```python
from build123d import *

# Parameters (mm, degrees)
SKETCH1_R               = 15
SKETCH1_R_2             = 3
BOSS_EXTRUDE1_DEPTH     = 10
SKETCH2_W               = 15
SKETCH2_H               = 30
BOSS_EXTRUDE2_DEPTH     = 10
FILLET1_R               = 15
SKETCH5_W               = 10
SKETCH5_H               = 2
BOSS_EXTRUDE3_DEPTH     = 10
BOSS_EXTRUDE4_START     = -3
SKETCH7_R               = 3
BOSS_EXTRUDE4_DEPTH     = 3
CHAMFER1_SIZE           = 0.7
BOSS_EXTRUDE6_DEPTH     = 10
FILLET4_R               = 2
FILLET2_R               = 10
CUT_EXTRUDE1_DEPTH      = 63.556116013
CUT_EXTRUDE1_DEPTH_BACK = 63.556116013
SKETCH10_R              = 1.25


with BuildPart() as part:
    # Sketch1 → Boss-Extrude1 (new body)
    with BuildSketch(Plane.XY):
        Circle(SKETCH1_R)
        Circle(SKETCH1_R_2, mode=Mode.SUBTRACT)
    extrude(amount=BOSS_EXTRUDE1_DEPTH)

    # Sketch2 → Boss-Extrude2 (add)
    with BuildSketch(Plane.XY):
        with Locations((0, 27.990381057)):
            Rectangle(SKETCH2_W, SKETCH2_H)
    extrude(amount=BOSS_EXTRUDE2_DEPTH)

    # Fillet1
    fillet1_edges = [part.edges().sort_by_distance(p)[0] for p in [
        (-7.5, 12.990381057, 5),
        (7.5, 12.990381057, 5),
    ]]
    fillet(fillet1_edges, radius=FILLET1_R)

    # Sketch5 → Boss-Extrude3 (add)
    with BuildSketch(Plane(origin=(0, 0, 0), x_dir=(-1, 0, 0), z_dir=(0, 0, -1))):
        with Locations((0, 2.5)):
            Rectangle(SKETCH5_W, SKETCH5_H)
    extrude(amount=-BOSS_EXTRUDE3_DEPTH)

    # Sketch7 → Boss-Extrude4 (add)
    with BuildSketch(Plane.XY.offset(10).offset(BOSS_EXTRUDE4_START)):
        Circle(SKETCH7_R)
    extrude(amount=BOSS_EXTRUDE4_DEPTH)

    # Chamfer1
    chamfer1_edges = [part.edges().sort_by_distance(p)[0] for p in [
        (0, 1.5, 7),
        (0, -3, 7),
    ]]
    chamfer(chamfer1_edges, length=CHAMFER1_SIZE)

    # Sketch9 → Boss-Extrude6 (add)
    with BuildSketch(Plane(origin=(0, 0, 0), x_dir=(-1, 0, 0), z_dir=(0, 0, -1))):
        with BuildLine():
            Line((-15, 53.990381057), (-15, 50.490381057))
            ThreePointArc((-15, 50.490381057), (-12.803300859, 45.187080198), (-7.5, 42.990381057))
            Line((-7.5, 42.990381057), (0, 42.990381057))
            Line((0, 42.990381057), (0, 46.490381057))
            Line((0, 46.490381057), (-7.5, 46.490381057))
            ThreePointArc((-7.5, 46.490381057), (-10.328427125, 47.661953932), (-11.5, 50.490381057))
            Line((-11.5, 50.490381057), (-11.5, 53.990381057))
            Line((-11.5, 53.990381057), (-15, 53.990381057))
        make_face()
        with BuildLine():
            Line((0, 46.490381057), (0, 42.990381057))
            Line((0, 42.990381057), (7.5, 42.990381057))
            ThreePointArc((7.5, 42.990381057), (12.803300859, 45.187080198), (15, 50.490381057))
            Line((15, 50.490381057), (15, 53.990381057))
            Line((15, 53.990381057), (11.5, 53.990381057))
            Line((11.5, 53.990381057), (11.5, 50.490381057))
            ThreePointArc((11.5, 50.490381057), (10.328427125, 47.661953932), (7.5, 46.490381057))
            Line((7.5, 46.490381057), (0, 46.490381057))
        make_face()
    extrude(amount=-BOSS_EXTRUDE6_DEPTH)

    # Fillet4
    # the kernel refuses this fillet: 2 mm, written as the material it takes off along each edge
    with BuildSketch(Plane(origin=(11.5, 53.990381057, -5), x_dir=(0, -1, 0), z_dir=(0, 0, 1)), Plane(origin=(15, 53.990381057, -5), x_dir=(-1, 0, 0), z_dir=(0, 0, 1)), Plane(origin=(-11.5, 53.990381057, -5), x_dir=(-1, 0, 0), z_dir=(0, 0, 1)), Plane(origin=(-15, 53.990381057, -5), x_dir=(0, -1, 0), z_dir=(0, 0, 1))) as fillet4_piece_1:
        with BuildLine():
            CenterArc((FILLET4_R, FILLET4_R), FILLET4_R, 180, 90)
            Line((0, FILLET4_R), (0, 0))
            Line((0, 0), (FILLET4_R, 0))
        make_face()
    extrude(amount=20, mode=Mode.SUBTRACT)

    # Fillet2
    fillet2_edges = [part.edges().sort_by_distance(p)[0] for p in [
        (-7.5, 42.990381057, 5),
        (7.5, 42.990381057, 5),
    ]]
    fillet(fillet2_edges, radius=FILLET2_R)

    # Sketch10 → Cut-Extrude1 (cut, two sides: drawn at the far end of the back side and taken through both)
    with BuildSketch(Plane(origin=(15, 0, 0), x_dir=(0, 0, -1), z_dir=(1, 0, 0)).offset(-CUT_EXTRUDE1_DEPTH_BACK)):
        with Locations((-5, 50.490381057)):
            Circle(SKETCH10_R)
    extrude(amount=CUT_EXTRUDE1_DEPTH + CUT_EXTRUDE1_DEPTH_BACK, mode=Mode.SUBTRACT)


solid = part.part
```
CAD build for the part. Positions are in the model's coordinates, mm. A direction names the side the tool comes from. Round coordinates to 2 decimals unless told otherwise and drop trailing zeros. Loops run counter-clockwise (first coordinate to the right, second up) from the corner with the lowest first, then second, coordinate; pieces in that order, holes last. Notation, with made-up numbers: M 50,-38 L 61,-38 A24 ccw 61,-14 Z; hole C -24,33 d10. An arc over 180 degrees is marked long. Use a Markdown table: item, result. Add a question column.
(1) Cut at C-C (y = 0). Give the cut face in (x, z).
(2) Cut at D-D (x = 0). Give the cut face in (y, z), and give its area (3 significant figures).
(3) Cut at B-B (x = 10.5). Give the cut face in (y, z).
(4) Cut at A-A (z = 2.75). Give the cut face in (x, y).
(5) Drill centre lines: line 1 (X direction, y = 50.5, z = 2.25); line 2 (Y direction, x = -13.65, z = 5); line 3 (Y direction, x = -13.85, z = 5). Where is each one in solid material? Low to high.
(6) Pull direction Y, two halves, no side cores. Call faces 1 (the face through (0, 46.49, 5)), 2 (the face through (0, 0, 7)), 3 (the face through (0, 12, 10)): +Y half, -Y half, draft (parallel to the pull), parting line (faces both ways), or undercut.
(7) Flat gauge pins, fed straight in: pin 1 (4 mm diameter, centred on x = -1, z = 4.5, fed in from -Y); pin 2 (2 mm diameter, centred on y = 50.49, z = 5, fed in from -X); pin 3 (1 mm diameter, centred on y = 20.5, z = 5, fed in from -X). Where does each tip first touch, or does it go through?
(8) Which spindle directions (+Z, -Z, +X, -X, +Y, -Y) get a long thin tool onto all of the face, cutting with end or side? Do faces 4 (the face through (0, 1.5, 3)), 5 (the face through (8.67, 40.82, 5.07)), 6 (the face through (-7.5, 28, 5)), 7 (the face through (10.297, 47.631, 4.93)). Say none if no direction does.
Geometry says:
| question | item | result |
|---|---|---|
| 1 | outline | M -15,0 L -3,0 L -3,6.3 L -2.3,7 L 2.3,7 L 3,6.3 L 3,0 L 15,0 L 15,10 L -15,10 Z |
| 2 | outline | M -15,0 L -3,0 L -3,6.3 L -2.3,7 L 0.8,7 L 1.5,6.3 L 1.5,0 L 46.49,0 L 46.49,10 L -15,10 Z |
| 2 | area | 584 mm² |
| 3 | outline | M -10.71,0 L 10.84,0 L 10.84,10 L -10.71,10 Z; M 43.27,0 L 47.84,0 L 47.84,10 L 43.27,10 Z |
| 4 | outline | M -15,50.49 A7.5 ccw -11.79,44.34 A10 cw -7.5,36.13 L -7.5,19.84 A15 cw -11.25,9.92 A15 ccw long 11.25,9.92 A15 cw 7.5,19.84 L 7.5,36.13 A10 cw 11.79,44.34 A7.5 ccw 15,50.49 L 15,51.99 A2 ccw 13.25,53.97 A2 ccw 11.5,51.99 L 11.5,50.49 A4 cw 7.5,46.49 L -7.5,46.49 A4 cw -11.5,50.49 L -11.5,51.99 A2 ccw -13.25,53.97 A2 ccw -15,51.99 Z; hole M -2.6,1.5 A3 ccw long 2.6,1.5 Z |
| 5 | line 1 | x = -15 to -11.5, 11.5 to 15 |
| 5 | line 2 | y = -6.22 to 6.22, 46.2 to 49.24, 51.74 to 53.88 |
| 5 | line 3 | y = -5.76 to 5.76, 46.5 to 49.24, 51.74 to 53.8 |
| 6 | face 1 | +Y half |
| 6 | face 2 | undercut |
| 6 | face 3 | draft |
| 7 | pin 1 | stops at y = -15 |
| 7 | pin 2 | passes through |
| 7 | pin 3 | stops at x = -7.5 |
| 8 | face 4 | -Z |
| 8 | face 5 | +Z, -Z, +X |
| 8 | face 6 | +Z, -Z, -X |
| 8 | face 7 | +Z, -Z, +Y |
